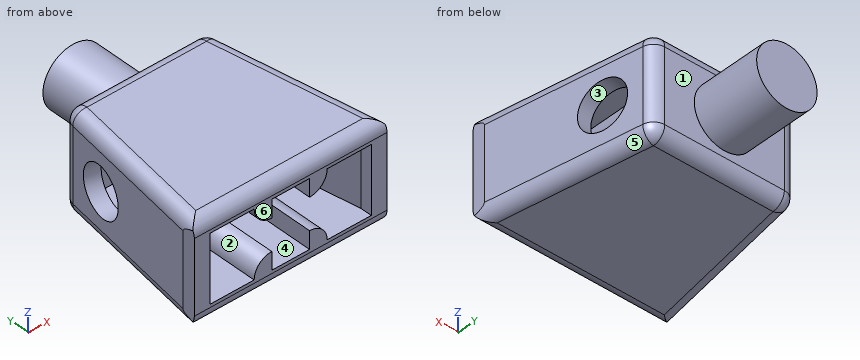
```python
from build123d import *

# Parameters (mm, degrees)
BOSS_EXTRUDE1_DEPTH  = 3.9
SHELL2_T             = -1.25
SKETCH5_R            = 1.9
CUT_EXTRUDE2_DEPTH   = 7.8
FILLET1_R            = 1
SKETCH6_R            = 2.4
BOSS_EXTRUDE2_DEPTH  = 5.5
SKETCH7_R            = 1.25
CUT_EXTRUDE3_DEPTH   = 4.25
BOSS_EXTRUDE3_DEPTH  = 12.449209595
MIRROR3_COPY_1_DEPTH = 12.449209595


with BuildPart() as part:
    # Sketch4 → Boss-Extrude1 (new, symmetric)
    with BuildSketch(Plane.XY):
        Polygon((7.65, 0), (-7.65, 0), (-7.65, 1), (-5.6, 13.699209595), (5.6, 13.699209595), (7.65, 1), align=None)
    extrude(amount=BOSS_EXTRUDE1_DEPTH, both=True)

    # Shell2
    shell2_openings = [part.faces().sort_by_distance(p)[0] for p in [
        (0, 0, 0),
    ]]
    offset(amount=SHELL2_T, openings=shell2_openings, kind=Kind.INTERSECTION)

    # Sketch5 → Cut-Extrude2 (cut)
    with BuildSketch(Plane(origin=(7.613040698, 1.228953134, 0), x_dir=(0, 0, -1), z_dir=(0.9872198433487761, 0.15936430245954739, 0))):
        with Locations(Location((0, 8.728225826, 0), (0, 0, 90))):
            Circle(SKETCH5_R)
    cut_extrude2 = extrude(amount=-CUT_EXTRUDE2_DEPTH, mode=Mode.SUBTRACT)

    # Mirror1: Cut-Extrude2 across plane
    add(cut_extrude2.mirror(Plane(origin=(0, 0, 0), x_dir=(0, 0, 1), z_dir=(1, 0, 0))), mode=Mode.SUBTRACT)

    # Fillet1
    # the kernel refuses this fillet: 1 mm, written as the material it takes off along each edge
    with BuildSketch(Plane(origin=(4.748481766, 12.699209595, -2.9), x_dir=(0, 1, 0), z_dir=(0, 0, -1))) as fillet1_piece_1_section:
        Polygon((0, 0), (FILLET1_R, 0), (FILLET1_R, FILLET1_R * 0.851518233962), (FILLET1_R * 0.15936430246, FILLET1_R * 0.987219843349), align=None)
    fillet1_piece_1 = extrude(amount=FILLET1_R, mode=Mode.PRIVATE)
    fillet1_piece_1 = fillet1_piece_1 - Plane(origin=(4.748481766, 12.699209595, -2.9), x_dir=(-0.6483192491128319, -0.7613686040478513, 0), z_dir=(0, 0, -1)) * Sphere(FILLET1_R, mode=Mode.PRIVATE)
    add(fillet1_piece_1, mode=Mode.SUBTRACT)
    with BuildSketch(Plane(origin=(4.748481766, 12.699209595, 2.9), x_dir=(0, 1, 0), z_dir=(0, 0, 1))) as fillet1_piece_2_section:
        Polygon((0, 0), (FILLET1_R, 0), (FILLET1_R, -FILLET1_R * 0.851518233962), (FILLET1_R * 0.15936430246, -FILLET1_R * 0.987219843349), align=None)
    fillet1_piece_2 = extrude(amount=FILLET1_R, mode=Mode.PRIVATE)
    fillet1_piece_2 = fillet1_piece_2 - Plane(origin=(4.748481766, 12.699209595, 2.9), x_dir=(-0.6483192491128319, -0.7613686040478513, 0), z_dir=(0, 0, 1)) * Sphere(FILLET1_R, mode=Mode.PRIVATE)
    add(fillet1_piece_2, mode=Mode.SUBTRACT)
    with BuildSketch(Plane(origin=(-4.748481766, 12.699209595, 2.9), x_dir=(-0.9872198433487762, 0.15936430245954666, 0), z_dir=(0, 0, 1))) as fillet1_piece_3_section:
        Polygon((0, 0), (FILLET1_R, 0), (FILLET1_R, -FILLET1_R * 0.851518233962), (FILLET1_R * 0.15936430246, -FILLET1_R * 0.987219843349), align=None)
    fillet1_piece_3 = extrude(amount=FILLET1_R, mode=Mode.PRIVATE)
    fillet1_piece_3 = fillet1_piece_3 - Plane(origin=(-4.748481766, 12.699209595, 2.9), x_dir=(0.6483192491128325, -0.7613686040478509, 0), z_dir=(0, 0, 1)) * Sphere(FILLET1_R, mode=Mode.PRIVATE)
    add(fillet1_piece_3, mode=Mode.SUBTRACT)
    with BuildSketch(Plane(origin=(-4.748481766, 12.699209595, -2.9), x_dir=(-0.9872198433487762, 0.15936430245954666, 0), z_dir=(0, 0, -1))) as fillet1_piece_4_section:
        Polygon((0, 0), (FILLET1_R, 0), (FILLET1_R, FILLET1_R * 0.851518233962), (FILLET1_R * 0.15936430246, FILLET1_R * 0.987219843349), align=None)
    fillet1_piece_4 = extrude(amount=FILLET1_R, mode=Mode.PRIVATE)
    fillet1_piece_4 = fillet1_piece_4 - Plane(origin=(-4.748481766, 12.699209595, -2.9), x_dir=(0.6483192491128325, -0.7613686040478509, 0), z_dir=(0, 0, -1)) * Sphere(FILLET1_R, mode=Mode.PRIVATE)
    add(fillet1_piece_4, mode=Mode.SUBTRACT)
    with BuildSketch(Plane(origin=(5.6, 13.699209595, -2.9), x_dir=(-1, 0, 0), z_dir=(0, 0, 1))) as fillet1_piece_5:
        with BuildLine():
            CenterArc((FILLET1_R * 0.851518233962, FILLET1_R), FILLET1_R, 189.17, 80.83)
            Line((-FILLET1_R * 0.135701609387, FILLET1_R * 0.84063569754), (0, 0))
            Line((0, 0), (FILLET1_R * 0.851518233962, 0))
        make_face()
    extrude(amount=5.8, mode=Mode.SUBTRACT)
    with BuildSketch(Plane(origin=(-4.748481766, 13.699209595, 3.9), x_dir=(0, -1, 0), z_dir=(1, 0, 0)), Plane(origin=(-4.748481766, 13.699209595, -3.9), x_dir=(0, 0, 1), z_dir=(1, 0, 0))) as fillet1_piece_6:
        with BuildLine():
            CenterArc((FILLET1_R, FILLET1_R), FILLET1_R, 180, 90)
            Line((0, FILLET1_R), (0, 0))
            Line((0, 0), (FILLET1_R, 0))
        make_face()
    extrude(amount=9.496963532, mode=Mode.SUBTRACT)
    with BuildSketch(Plane(origin=(-5.6, 13.699209595, 2.9), x_dir=(-0.15936430245954636, -0.9872198433487762, 0), z_dir=(0, 0, -1))) as fillet1_piece_7:
        with BuildLine():
            CenterArc((FILLET1_R * 0.851518233962, -FILLET1_R), FILLET1_R, 90, 80.83)
            Line((-FILLET1_R * 0.135701609387, -FILLET1_R * 0.84063569754), (0, 0))
            Line((0, 0), (FILLET1_R * 0.851518233962, 0))
        make_face()
    extrude(amount=5.8, mode=Mode.SUBTRACT)
    with BuildSketch(Plane(origin=(5.735701609, 12.858573897, 3.9), x_dir=(-0.9872198433487762, -0.15936430245954736, 0), z_dir=(0.15936430245954736, -0.9872198433487761, 0)), Plane(origin=(5.735701609, 12.858573897, -3.9), x_dir=(0, 0, 1), z_dir=(0.15936430245954736, -0.9872198433487761, 0)), Plane(origin=(-8.048410756, -1.468049608, -3.9), x_dir=(0, 0, 1), z_dir=(0.15936430245954666, 0.9872198433487762, 0)), Plane(origin=(-8.048410756, -1.468049608, 3.9), x_dir=(0.9872198433487762, -0.15936430245954664, 0), z_dir=(0.15936430245954666, 0.9872198433487762, 0))) as fillet1_piece_8:
        with BuildLine():
            CenterArc((FILLET1_R, FILLET1_R), FILLET1_R, 180, 90)
            Line((0, FILLET1_R), (0, 0))
            Line((0, 0), (FILLET1_R, 0))
        make_face()
    extrude(amount=14.512090293, mode=Mode.SUBTRACT)
    with BuildSketch(Plane(origin=(10.15, 0, 3.9), x_dir=(0, 1, 0), z_dir=(-1, 0, 0)), Plane(origin=(10.15, 0, -3.9), x_dir=(0, 0, 1), z_dir=(-1, 0, 0))) as fillet1_piece_9:
        with BuildLine():
            CenterArc((FILLET1_R, FILLET1_R), FILLET1_R, 180, 90)
            Line((0, FILLET1_R), (0, 0))
            Line((0, 0), (FILLET1_R, 0))
        make_face()
    extrude(amount=20.3, mode=Mode.SUBTRACT)

    # Sketch6 → Boss-Extrude2 (add)
    with BuildSketch(Plane(origin=(0, 13.699209595, 0), x_dir=(1, 0, 0), z_dir=(0, 1, 0))):
        Circle(SKETCH6_R)
    extrude(amount=BOSS_EXTRUDE2_DEPTH)

    # Sketch7 → Cut-Extrude3 (cut)
    with BuildSketch(Plane.XZ.offset(-12.449209595)):
        Circle(SKETCH7_R)
    extrude(amount=-CUT_EXTRUDE3_DEPTH, mode=Mode.SUBTRACT)

    # Sketch8 → Boss-Extrude3 (add)
    with BuildSketch(Plane.XZ):
        with BuildLine():
            Line((-1.5, -2.65), (-1.5, -1.25))
            ThreePointArc((-1.5, -1.25), (-2.489949494, -1.660050506), (-2.9, -2.65))
            Line((-2.9, -2.65), (-1.5, -2.65))
        make_face()
    boss_extrude3 = extrude(amount=-BOSS_EXTRUDE3_DEPTH)

    # Mirror2: Boss-Extrude3 across plane
    add(boss_extrude3.mirror(Plane(origin=(0, 0, 0), x_dir=(0, 0, 1), z_dir=(1, 0, 0))))

    # Mirror3: Boss-Extrude3 across plane
    add(boss_extrude3.mirror(Plane.XY))

    # Mirror3 copy 1 sketch → Mirror3 copy 1 (add)
    with BuildSketch(Plane(origin=(0, 0, 0), x_dir=(-1, 0, 0), z_dir=(0, -1, 0))):
        with BuildLine():
            Line((-1.5, -2.65), (-1.5, -1.25))
            ThreePointArc((-1.5, -1.25), (-2.489949494, -1.660050506), (-2.9, -2.65))
            Line((-2.9, -2.65), (-1.5, -2.65))
        make_face()
    extrude(amount=-MIRROR3_COPY_1_DEPTH)


solid = part.part
```
CAD build for the part. Positions are in the model's coordinates, mm. Face numbers are marked on the shaded views. A direction names the side the tool comes from. Round coordinates to 2 decimals unless told otherwise and drop trailing zeros. Order: outer loops, then holes, each group sorted by start corner. A loop starts at its lowest first (then second) coordinate and runs counter-clockwise, first axis right, second up.
Item 1: Saw through at A-A on x = 3.5. Write the cut outline in (y, z), then the cut area to 3 significant figures.
Item 2: Saw through at D-D on x = 0. Write the cut outline in (y, z), then the cut area to 3 significant figures.
Item 3: Saw through at B-B on z = 0. State how many separate pieces and enclosed holes the cut face has, then the cut area to 3 significant figures.
Item 4: Saw through at C-C on y = 15.5. Write the cut outline in (x, z).
Item 5: Pin check, flat tips, straight feed: pin 1 (1.1 mm diameter, centred on y = 7.5, z = -2, fed in from +X); pin 2 (2 mm diameter, centred on x = 0, z = 0, fed in from -Y); pin 3 (1 mm diameter, centred on y = 2, z = -0.5, fed in from +X). Stop position of each tip, or through.
Item 6: Tool access for the marked faces 1, 2 and 3: list every direction of +Z, -Z, +X, -X, +Y, -Y with a clear straight run to the whole face (end or side of a thin tool).
Item 7: Mould opens along X. For the marked faces 4, 5 and 6 say: pulls with the +X half, pulls with the -X half, needs draft (parallel to the pull), parting line crosses it, or undercut.
Item 8: Probe line 1 along Z through (x, y) = (0, 14.05); line 2 along Y through (x, z) = (1.5, 0.5); line 3 along Z through (x, y) = (3, 1.25). List the from-to ranges inside material, lowest first.
Reported:
1. outline: (0, -2.9) arc R1 ccw to (1, -3.9) - (12.7, -3.9) arc R1 ccw to (13.7, -2.9) - (13.7, 2.9) arc R1 ccw to (12.7, 3.9) - (1, 3.9) arc R1 ccw to (0, 2.9) - (0, 2.65) - (12.45, 2.65) - (12.45, -2.65) - (0, -2.65) - close
1. area: 40.0 mm2
2. outline: (0, -2.9) arc R1 ccw to (1, -3.9) - (12.7, -3.9) arc R1 ccw to (13.7, -2.9) - (13.7, -2.4) - (19.2, -2.4) - (19.2, 2.4) - (13.7, 2.4) - (13.7, 2.9) arc R1 ccw to (12.7, 3.9) - (1, 3.9) arc R1 ccw to (0, 2.9) - (0, 2.65) - (12.45, 2.65) - (12.45, 1.25) - (16.7, 1.25) - (16.7, -1.25) - (12.45, -1.25) - (12.45, -2.65) - (0, -2.65) - close
2. area: 55.8 mm2
3. separate pieces: 3
3. enclosed holes: 0
3. area: 51.7 mm2
4. outline: circle Ø4.8 at (0, 0); hole circle Ø2.5 at (0, 0)
5. pin 1: stops at x = 6.69
5. pin 2: stops at y = 16.7
5. pin 3: stops at x = 7.57
6. face 1: +Y
6. face 2: -Y
6. face 3: none
7. face 4: undercut
7. face 5: pulls with the +X half
7. face 6: needs draft
8. line 1: z = -2.4 to -1.25, 1.25 to 2.4
8. line 2: y = 12.45 to 19.2
8. line 3: z = -3.9 to -2.65, 2.65 to 3.9
